from build123d import *

# Parameters (mm, degrees)
F1_R     = 1.5
F2_DEPTH = 20
F3_W     = 2
F3_H     = 7
F4_DEPTH = 25
F5_W     = 9.7
F5_H     = 11.5
F6_DEPTH = 25


# Not quite as in the source:
# - ends of sketch curves that miss each other by under 0.0002 mm in the source are joined


with BuildPart() as f2:
    # F1 (on Front) → F2 (new body)
    with BuildSketch(Plane.XZ):
        with BuildLine():
            Line((-22.3164947392, 83.8837339027), (-17.7874447277, 79.2521323433))
            ThreePointArc((-17.7874447277, 79.2521323433), (-14.2521323433, 79.2125552723), (-14.2125552723, 82.7478676567))
            Line((-14.2125552723, 82.7478676567), (-18.9921983086, 87.6357364337))
            Line((-18.9921983086, 87.6357364337), (-17.5868240881, 87.8835418245))
            Line((-17.5868240881, 87.8835418245), (-14.5868240881, 88.4125227619))
            Line((-14.5868240881, 88.4125227619), (0, 90.9845733884))
            Line((0, 90.9845733884), (0, 92))
            Line((0, 92), (-21.474961, 88.213385))
            ThreePointArc((-21.474961, 88.213385), (-22.6081005709, 87.5885032671), (-23.1214986845, 86.4006879752))
            Line((-23.1214986845, 86.4006879752), (-24.456969, 69.431938))
            ThreePointArc((-24.456969, 69.431938), (-24.4963407526, 69.1645008146), (-24.5714176946, 68.9048158888))
            Line((-24.5714176946, 68.9048158888), (-33.651464, 43.957595))
            ThreePointArc((-33.651464, 43.957595), (-33.757171385, 43.0298159786), (-33.4301544738, 42.1551686804))
            Line((-33.4301544738, 42.1551686804), (-25.341925, 30.163876))
            ThreePointArc((-25.341925, 30.163876), (-25.0873905233, 29.6302335248), (-25, 29.04549))
            Line((-25, 29.04549), (-25, 27))
            Line((-25, 27), (-25, -0.5))
            Line((-25, -0.5), (-24.0000002534, -0.5))
            Line((-24.0000002534, -0.5), (-24.0000002534, 27))
            Line((-24.0000002534, 27), (-17, 27))
            ThreePointArc((-17, 27), (-14.5, 29.5), (-17, 32))
            Line((-17, 32), (-25, 32))
            Line((-25, 32), (-25.3741885909, 32))
            Line((-25.3741885909, 32), (-32.6011163068, 42.7143612935))
            ThreePointArc((-32.6011163068, 42.7143612935), (-32.7646248248, 43.1516847064), (-32.7117713086, 43.6155740346))
            Line((-32.7117713086, 43.6155740346), (-23.6317251212, 68.5627955495))
            ThreePointArc((-23.6317251212, 68.5627955495), (-23.5191096678, 68.9523229367), (-23.4600509821, 69.3534786388))
            Line((-23.4600509821, 69.3534786388), (-22.5711850089, 80.6475881907))
            Line((-22.5711850089, 80.6475881907), (-22.3164947392, 83.8837339027))
        make_face()
        with Locations((-17, 29.5)):
            Circle(F1_R, mode=Mode.SUBTRACT)
        with Locations((-16, 81)):
            Circle(F1_R, mode=Mode.SUBTRACT)
        with BuildLine():
            Line((-24.0000002534, -28), (-24.0000002534, -0.5))
            Line((-24.0000002534, -0.5), (-25, -0.5))
            Line((-25, -0.5), (-25, -30.04549))
            ThreePointArc((-25, -30.04549), (-25.0873905233, -30.6302335248), (-25.3419249898, -31.1638760069))
            Line((-25.341925, -31.163876), (-26.5804062367, -33))
            Line((-26.5804062367, -33), (-25, -33))
            Line((-25, -33), (-17, -33))
            ThreePointArc((-17, -33), (-14.5, -30.5), (-17, -28))
            Line((-17, -28), (-24.0000002534, -28))
        make_face()
        with Locations((-17, -30.5)):
            Circle(F1_R, mode=Mode.SUBTRACT)
    extrude(amount=F2_DEPTH)

    # F3 (on face) → F4 (cut)
    with BuildSketch(Plane(origin=(-43.8426892635, 0, 15.9574341077), x_dir=(0, -1, 0), z_dir=(-0.9396926192, 0, 0.3420201476))):
        with Locations((1, 37.1150750518)):
            Rectangle(F3_W, F3_H)
    extrude(amount=-F4_DEPTH, mode=Mode.SUBTRACT)

    # F5 (on face) → F6 (cut)
    with BuildSketch(Plane(origin=(-25, 0, 0), x_dir=(0, -1, 0), z_dir=(-1, 0, 0))):
        with Locations((6.8, -0.5)):
            Rectangle(F5_W, F5_H)
    extrude(amount=-F6_DEPTH, mode=Mode.SUBTRACT)


solid = f2.part
For this review, take the finished solid that the model builds, in its own axes (mm). A direction names the side the tool comes from. Round coordinates to 2 decimals unless told otherwise and drop trailing zeros. Loops run counter-clockwise (first coordinate to the right, second up) from the corner with the lowest first, then second, coordinate; pieces in that order, holes last. Notation, with made-up numbers: (89, 83.25) - (130, 83.25) arc R28 cw to (130, 111.25) - close; hole circle Ø11 at (33.5, 37.25). An arc over 180 degrees is marked (long way). Use one line per item in the form item = value.
Item 1: Tool access review of faces 1 (the flat face through (-16.57, -9.86, 85.16)), 2 (the flat face through (-22, -10, -33)): name each direction out of +Z, -Z, +X, -X, +Y, -Y from which nothing blocks a thin tool from reaching the whole face with its end or side.
Answers:
face_1 = +X, +Y, -Y
face_2 = -Z, +X, -X, +Y, -Y
Item 2: For line 1 (X direction, y = -1.5, z = 80.5); line 2 (X direction, y = -8.25, z = 81); line 3 (X direction, y = -6, z = 6.5), list the stretches that pass through material, from the lowest coordinate up.
Answers:
line_1 = -23.59 to -22.58, -19.01 to -17.41, -14.59 to -13.55
line_2 = -23.55 to -22.54, -19.5 to -17.5, -14.5 to -13.5
line_3 = -25 to -24
Item 3: Consider section C-C on z = -10.5. Write out the cut boundary in (x, y).
Answers:
outline = (-25, -20) - (-24, -20) - (-24, 0) - (-25, 0) - close
Item 4: Clearance check with flat-ended pins moving along their axes: P1, Ø1.8, axis at x = -16, z = 81, coming from the +Y side; P2, Ø3.5, axis at x = -21.5, y = -9, coming from the +Z side; P3, Ø10, axis at y = -5, z = 14.5, coming from the +X side; P4, Ø2.5, axis at x = -23, y = -6, coming from the +Z side. State where each tip first meets the part, or that it passes through.
Answers:
P1 = through
P2 = 88.52
P3 = -24
P4 = 88.14
Item 5: Mouldability with a two-part tool opening along X and no side actions: class faces 3 (the flat face through (-20, -10, -28)), 4 (the cylindrical face through (-18.11, -9.86, 30.51)), 5 (the cylindrical face through (-14.5, -9.9, -30.6)) as +X half, -X half, draft (parallel to the pull), parting line (faces both ways), or undercut.
Answers:
face_3 = draft
face_4 = undercut
face_5 = +X half
Item 6: Consider section D-D on x = -11.5. Write out the cut boundary in (y, z), then the cut area to 3 significant figures.
Answers:
outline = (-20, 88.96) - (0, 88.96) - (0, 89.97) - (-20, 89.97) - close
area = 20.3 mm^2
Item 7: Consider section A-A on y = -13.5. State how many separate pieces and enclosed holes the cut face has, then the cut area to 3 significant figures.
Answers:
separate_pieces = 1
enclosed_holes = 3
area = 267 mm^2
